```python
from build123d import *

# Parameters (mm, degrees)
F3_DEPTH = 1.5875
F2_W     = 12.7
F2_H     = 3.175
F4_DEPTH = 12.7
F1_R     = 1.5875
F5_DEPTH = 12.7


with BuildPart() as f3:
    # F0 (on Right) → F3 (new body, symmetric)
    with BuildSketch(Plane.YZ):
        with BuildLine():
            Line((-56.068145, 20.917505), (-25.4, 12.7))
            Line((-25.4, 12.7), (25.4, 12.7))
            Line((25.4, 12.7), (25.4, 44.45))
            ThreePointArc((25.4, 44.45), (22.225, 47.625), (19.05, 44.45))
            Line((19.05, 44.45), (19.05, 22.225))
            Line((19.05, 22.225), (-24.14601, 22.225))
            Line((-24.14601, 22.225), (-53.602894, 30.117948))
            ThreePointArc((-53.602894, 30.117948), (-59.435741, 26.750352), (-56.068145, 20.917505))
        make_face()
    extrude(amount=F3_DEPTH, both=True)

    # F2 (on Right) → F4 (cut, symmetric)
    with BuildSketch(Plane.YZ):
        with Locations((6.35, 22.225)):
            Rectangle(F2_W, F2_H)
    extrude(amount=F4_DEPTH, both=True, mode=Mode.SUBTRACT)

    # F1 (on Right) → F5 (cut, symmetric)
    with BuildSketch(Plane.YZ):
        with Locations((-54.835519, 25.517726)):
            Circle(F1_R)
    extrude(amount=F5_DEPTH, both=True, mode=Mode.SUBTRACT)


solid = f3.part
```
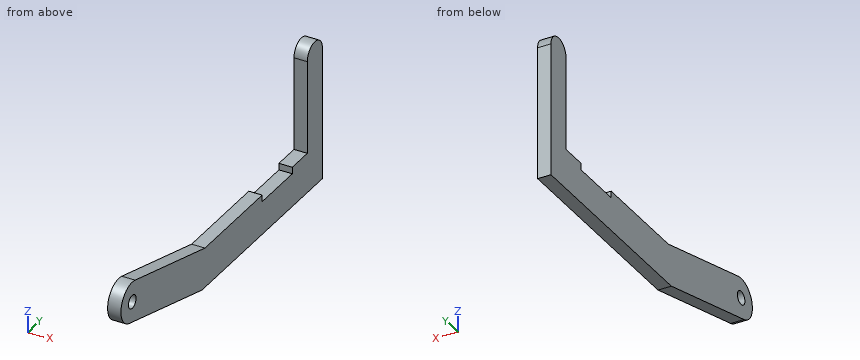
The model under review builds one solid part; all positions refer to its coordinate system, in mm. Give positions to 0.01 mm unless a question says otherwise; leave off trailing zeros. Write each loop counter-clockwise with the first axis right and the second up, starting at its lowest first coordinate (ties: lowest second). Pieces come first, ordered by that corner, then holes. Notation, with made-up numbers: M -0.75,-36 L 17.25,-36 A27 ccw 17.25,3 Z; hole C 58,29.5 d3. An arc over 180 degrees is marked long. Write item = value, one per line. Start each with the question number.
Q1. We need section C-C (z = 37). State the section outline as (x, y) points, plus the area to 3 significant figures.
Q2. Clearance check with flat-ended pins moving along their axes: pin 1 (1 mm diameter, centred on x = -0.5, y = 5, fed in from +Z); pin 2 (1 mm diameter, centred on x = 0.5, y = -16, fed in from +Z) (3 decimals); pin 3 (1.3 mm diameter, centred on x = -0.5, z = 21.5, fed in from -Y). State where each tip first meets the part, or that it passes through.
Q3. For line 1 (Y direction, x = -0.5, z = 41.5); line 2 (Z direction, x = 1.35, y = -2.5) (3 decimals), list the stretches that pass through material, from the lowest coordinate up.
Q4. We need section B-B (y = 6.5). State the section outline as (x, z) points, plus the area to 3 significant figures.
Result set:
q1.outline = M -1.59,19.05 L 1.59,19.05 L 1.59,25.4 L -1.59,25.4 Z
q1.area = 20.2 mm2
q2.pin_1 = 20.64
q2.pin_2 = 22.225
q2.pin_3 = -58.2
q3.line_1 = 19.05 to 25.4
q3.line_2 = 12.7 to 22.225
q4.outline = M -1.59,12.7 L 1.59,12.7 L 1.59,20.64 L -1.59,20.64 Z
q4.area = 25.2 mm2
